from build123d import *

# Parameters (mm, degrees)
BOSS_EXTRUDE1_DEPTH = 1


with BuildPart() as part:
    # Sketch2 → Boss-Extrude1 (new, symmetric)
    with BuildSketch(Plane.XY):
        with BuildLine():
            Line((30, 0), (95, 0))
            Line((95, 0), (95, 230))
            Line((95, 230), (4, 230))
            Line((4, 230), (3.430566833, 235))
            Line((3.430566833, 235), (3.430566833, 240))
            Line((3.430566833, 240), (-3.430566833, 240))
            Line((-3.430566833, 240), (-3.430566833, 235))
            Line((-3.430566833, 235), (-4, 230))
            Line((-4, 230), (-95, 230))
            Line((-95, 230), (-95, 0))
            Line((-95, 0), (-30, 0))
            ThreePointArc((-30, 0), (0, 30), (30, 0))
        make_face()
    extrude(amount=BOSS_EXTRUDE1_DEPTH, both=True)


solid = part.part
The model under review builds one solid part; all positions refer to its coordinate system, in mm. Give positions to 0.01 mm unless a question says otherwise; leave off trailing zeros. Order: outer loops, then holes, each group sorted by start corner. A loop starts at its lowest first (then second) coordinate and runs counter-clockwise, first axis right, second up. Notation, with made-up numbers: M 42.25,77 L 77.25,77 A21 cw 77.25,98 Z; hole C 50,-27.75 d3. An arc over 180 degrees is marked long. Answer in a Markdown table with one row per item. Add a question column.
1. Add section C-C on x = -43. State the section outline as (y, z) points.
2. For pin 1 Ø0.6 at (y, z) = (238.5, 0) entering from -X; pin 2 Ø1 at (x, z) = (73, 0) entering from +Y, all flat-tipped, find the tip position at first contact; note any pin that passes through.
3. Add section B-B on y = 17.5. State the section outline as (x, z) points, plus the area to 3 significant figures.
4. Add section D-D on x = 0. State the section outline as (y, z) points.
5. Mouldability with a two-part tool opening along X and no side actions: class faces 1 (the flat face through (-1, 122, -1)), 2 (the cylindrical face through (-0.66, 29.993, 0.014)) as released by +X, released by -X, zero draft, split by the parting line, or undercut.
6. To check wall thickness, follow line 1 along Y through (x, z) = (-58, -0.25); line 2 along X through (y, z) = (21, -0.25); line 3 along X through (y, z) = (12.5, 0.3). State the ranges of each line that lie inside material, in increasing order.
7. Add section A-A on z = -0.45. State the section outline as (x, y) points.
The answers:
| question | item | result |
|---|---|---|
| 1 | outline | M 0,-1 L 230,-1 L 230,1 L 0,1 Z |
| 2 | pin 1 | x = -3.43 |
| 2 | pin 2 | y = 230 |
| 3 | outline | M -95,-1 L -24.37,-1 L -24.37,1 L -95,1 Z; M 24.37,-1 L 95,-1 L 95,1 L 24.37,1 Z |
| 3 | area | 283 mm2 |
| 4 | outline | M 30,-1 L 240,-1 L 240,1 L 30,1 Z |
| 5 | face 1 | zero draft |
| 5 | face 2 | undercut |
| 6 | line 1 | 0 to 230 |
| 6 | line 2 | -95 to -21.42, 21.42 to 95 |
| 6 | line 3 | -95 to -27.27, 27.27 to 95 |
| 7 | outline | M -95,0 L -30,0 A30 cw 30,0 L 95,0 L 95,230 L 4,230 L 3.43,235 L 3.43,240 L -3.43,240 L -3.43,235 L -4,230 L -95,230 Z |
